```python
from build123d import *

# Parameters (mm, degrees)
RESSALTO_EXTRUS_O1_DEPTH = 5
ESBO_O2_R                = 1.5
CORTE_EXTRUS_O1_DEPTH    = 10
ESBO_O3_R                = 1.5
CORTE_EXTRUS_O2_DEPTH    = 6


with BuildPart() as part:
    # Esboço1 → Ressalto-extrusão1 (new body)
    with BuildSketch(Plane.XY):
        with BuildLine():
            Line((44.495405461, -168.430491325), (44.495405461, -144.332190763))
            Line((44.495405461, -144.332190763), (-55.573351401, -144.332190763))
            Line((-55.573351401, -144.332190763), (-55.573351401, -168.393072388))
            Line((-55.573351401, -168.393072388), (-55.504594539, -168.430491325))
            ThreePointArc((-55.504594539, -168.430491325), (-5.504594539, -299.332190763), (44.495405461, -168.430491325))
        make_face()
    extrude(amount=RESSALTO_EXTRUS_O1_DEPTH)

    # Esboço2 → Corte-extrusão1 (cut)
    with BuildSketch(Plane.XY.offset(5)):
        with Locations((39.44625518, -173.430491325)):
            Circle(ESBO_O2_R)
        with Locations((52.44625518, -187.430491325)):
            Circle(ESBO_O2_R)
        with Locations((54.44625518, -258.430491325)):
            Circle(ESBO_O2_R)
        with Locations((-13.455444258, -293.430491325)):
            Circle(ESBO_O2_R)
        with Locations((2.44625518, -293.430491325)):
            Circle(ESBO_O2_R)
        with Locations((-65.455444258, -258.430491325)):
            Circle(ESBO_O2_R)
        with Locations((-63.455444258, -187.430491325)):
            Circle(ESBO_O2_R)
        with Locations((-50.455444258, -173.430491325)):
            Circle(ESBO_O2_R)
    extrude(amount=-CORTE_EXTRUS_O1_DEPTH, mode=Mode.SUBTRACT)

    # Esboço3 → Corte-extrusão2 (cut, through all)
    with BuildSketch(Plane.XY.offset(5)):
        with Locations((-53.073351401, -162.430491325)):
            Circle(ESBO_O3_R)
        with Locations((-53.073351401, -155.332190763)):
            Circle(ESBO_O3_R)
        with Locations((41.995405461, -162.430491325)):
            Circle(ESBO_O3_R)
        with Locations((41.995405461, -155.332190763)):
            Circle(ESBO_O3_R)
    extrude(amount=-CORTE_EXTRUS_O2_DEPTH, mode=Mode.SUBTRACT)


solid = part.part
```
The model under review builds one solid part; all positions refer to its coordinate system, in mm. A direction names the side the tool comes from. Round coordinates to 2 decimals unless told otherwise and drop trailing zeros. Order: outer loops, then holes, each group sorted by start corner. A loop starts at its lowest first (then second) coordinate and runs counter-clockwise, first axis right, second up.
(1) Take a section at B-B, the plane y = -210.5. State the section outline as (x, z) points, plus the area to 3 significant figures.
Working result:
outline: (-79.22, 0) - (68.21, 0) - (68.21, 5) - (-79.22, 5) - close
area: 737 mm2
(2) Take a section at C-C, the plane x = 60.5. State the section outline as (y, z) points.
Working result:
outline: (-259.95, 0) - (-188.72, 0) - (-188.72, 5) - (-259.95, 5) - close
(3) Wall thickness on L1, parallel to X at y = -187, z = 1.3; L2, parallel to X at y = -222.5, z = 4.05; L3, parallel to Y at x = 43, z = 3.05: over which ranges is each line inside the solid? List them lowest first.
Working result:
L1: x = -70.55 to -64.89, -62.02 to 51.01, 53.88 to 59.54
L2: x = -80.48 to 69.47
L3: y = -281.54 to -163.54, -161.32 to -156.45, -154.22 to -144.33
(4) For P1, Ø1, axis at x = 16.5, y = -181, coming from the -Z side; P2, Ø1, axis at y = -190.5, z = 0.5, coming from the -X side, all flat-tipped, find the tip position at first contact; note any pin that passes through.
Working result:
P1: stops at z = 0
P2: stops at x = -72.69
(5) Take a section at A-A, the plane z = 1.45. Count the separate pieces of the cut face and the enclosed holes in it, plus the area to 3 significant figures.
Working result:
separate pieces: 1
enclosed holes: 12
area: 18,700 mm2
(6) Tool access review of faces 1 (the face through (-55.573, -156, 2)), 2 (the face through (-7, -221, 0)), 3 (the face through (44.495, -157, 2)): name each direction out of +Z, -Z, +X, -X, +Y, -Y from which nothing blocks a thin tool from reaching the whole face with its end or side.
Working result:
face 1: +Z, -Z, -X, +Y
face 2: -Z, +X, -X, +Y, -Y
face 3: +Z, -Z, +X, +Y
